Verification items for the finished model (mm, model axes). Face numbers are marked on the shaded views. Coordinates: 2 decimals unless noted, no trailing zeros. Loops run counter-clockwise (first coordinate to the right, second up) from the corner with the lowest first, then second, coordinate; pieces in that order, holes last. Notation, with made-up numbers: (79, -9) - (116, -9) arc R18 ccw to (116, 6) - close; hole circle Ø4 at (59.25, -9). An arc over 180 degrees is marked (long way). One line per item, written item: value. Start each with the question number.
(1) Thickness scan on probe 1 along Y at (x, z) = (-50.5, 13.5); probe 2 along Y at (x, z) = (-138, 17); probe 3 along Z at (x, y) = (-50, -505.5). Record the ranges inside material, lowest first. Write a range as [from, to].
(2) Draft check along X on the marked faces 1 and 2. Enter one of: +X half, -X half, draft (parallel to the pull), parting line (faces both ways), or undercut.
(3) Section check B-B (x = -124). Record the boundary of the cut face in (y, z), plus the area to 3 significant figures.
(4) Section check A-A (y = -171.5). Record the boundary of the cut face in (x, z), plus the area to 3 significant figures.
(5) Gauge pin test, flat ends, axial feed: P1, Ø6, axis at y = -62, z = 20, coming from the -X side; P2, Ø8, axis at x = 48.5, y = 283, coming from the -Z side; P3, Ø6, axis at x = 187.5, z = 12.56, coming from the +Y side. Record the tip position at first contact, or that the pin passes through.
```python
from build123d import *

# Parameters (mm, degrees)
F0_W     = 410
F0_H     = 1028
F1_DEPTH = 25
F2_R     = 5
F3_DEPTH = 14
F4_R     = 5
F5_DEPTH = 14
F7_DEPTH = 1028
F8_W     = 310
F8_H     = 940
F9_DEPTH = 19


with BuildPart() as f1:
    # F0 (on Top) → F1 (new body)
    with BuildSketch(Plane.XY):
        Rectangle(F0_W, F0_H)
    extrude(amount=F1_DEPTH)

    # F2 (on face) → F3 (cut)
    with BuildSketch(Plane.XZ.offset(514)):
        with Locations((187.5, 12.5)):
            Circle(F2_R)
        with Locations((-50, 12.5)):
            Circle(F2_R)
    extrude(amount=-F3_DEPTH, mode=Mode.SUBTRACT)

    # F4 (on face) → F5 (cut)
    with BuildSketch(Plane(origin=(0, 514, 0), x_dir=(-1, 0, 0), z_dir=(0, 1, 0))):
        with Locations((-187.5, 12.5625)):
            Circle(F4_R)
        with Locations((50, 12.5625)):
            Circle(F4_R)
    extrude(amount=-F5_DEPTH, mode=Mode.SUBTRACT)

    # F6 (on face) → F7 (join)
    with BuildSketch(Plane.XZ.offset(514)):
        with BuildLine():
            Line((-205, 0.342944), (-205, 25))
            Line((-205, 25), (-230.672767, 25))
            ThreePointArc((-230.672767, 25), (-232.082307, 24.013028), (-231.636945, 22.350931))
            Line((-231.636945, 22.350931), (-206.394084, 1.169769))
            ThreePointArc((-206.394084, 1.169769), (-205.730769, 0.699491), (-205, 0.342944))
        make_face()
    extrude(amount=-F7_DEPTH)

    # F8 (on face) → F9 (cut)
    with BuildSketch(Plane(origin=(0, 0, 0), x_dir=(1, 0, 0), z_dir=(0, 0, -1))):
        with Locations((0, -4)):
            Rectangle(F8_W, F8_H)
    extrude(amount=-F9_DEPTH, mode=Mode.SUBTRACT)


solid = f1.part
```
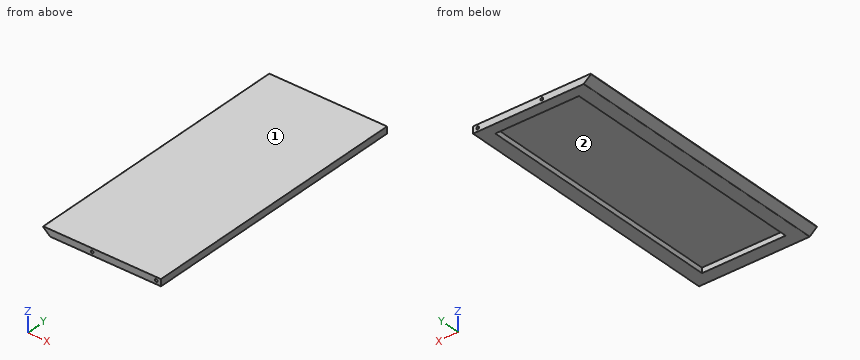
Responses:
1. probe 1: y = [-500, -466], [474, 500]
1. probe 2: y = [-514, -466], [474, 514]
1. probe 3: z = [0, 7.5], [17.5, 25]
2. face 1: draft
2. face 2: undercut
3. outline: (-514, 0) - (-466, 0) - (-466, 19) - (474, 19) - (474, 0) - (514, 0) - (514, 25) - (-514, 25) - close
3. area: 7,840 mm²
4. outline: (-231.64, 22.35) - (-206.39, 1.17) arc R5 ccw to (-205, 0.34) - (-205, 0) - (-155, 0) - (-155, 19) - (155, 19) - (155, 0) - (205, 0) - (205, 25) - (-230.67, 25) arc R1.5 ccw to start
4. area: 4,730 mm²
5. P1: stops at x = -232.09
5. P2: stops at z = 19
5. P3: stops at y = 500
